Job drawing, mm, ordinate dimensions from the low corner. One solid piece. A direction names the side the tool comes from. Give positions to 0.01 mm unless a question says otherwise; leave off trailing zeros. Order: outer loops, then holes, each group sorted by start corner. A loop starts at its lowest first (then second) coordinate and runs counter-clockwise, first axis right, second up.
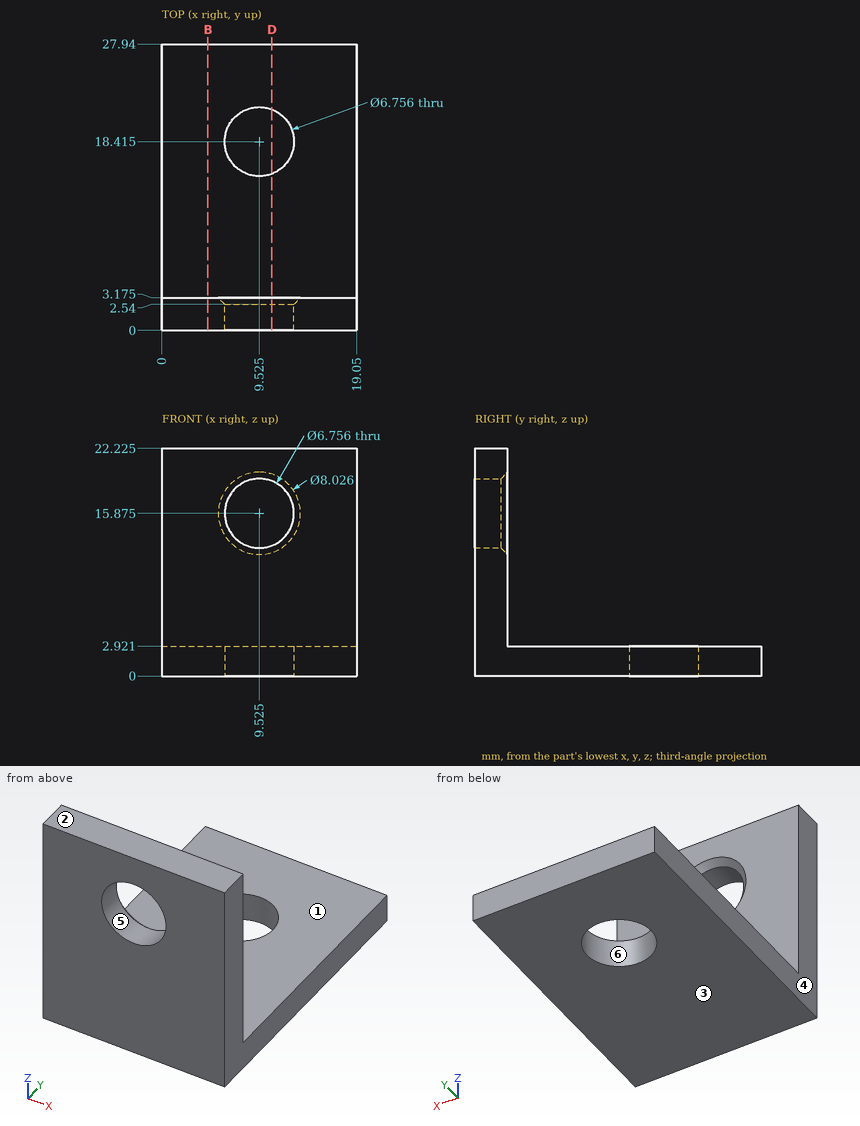
Item 1: Pull direction X, two halves, no side cores. Call the marked faces 3, 4, 5 and 6: released by +X, released by -X, zero draft, split by the parting line, or undercut.
Item 2: Drill centre lines: probe 1 along Z at (x, y) = (17, 18.75); probe 2 along Y at (x, z) = (1.5, 6) (1 decimal); probe 3 along X at (y, z) = (2.5, 13.5). Where is each one in solid material? Low to high.
Item 3: Drop flat-ended pins along their axis: P1, Ø4, axis at x = 4.5, y = 9, coming from the +Z side; P2, Ø6, axis at x = 9.525, y = 18.415, coming from the +Z side. Give the stop position or say it passes through.
Item 4: Band-saw the part on D-D on x = 10.75. Give the number of separate pieces and of enclosed holes in the cut face, plus the area to 3 significant figures.
Item 5: Which spindle directions (+Z, -Z, +X, -X, +Y, -Y) get a long thin tool onto all of the face, cutting with end or side? Do the marked faces 1 and 2. Say none if no direction does.
Item 6: Band-saw the part on B-B on x = 4.5. List the corners of the cut face in (y, z) (1 decimal), plus the area to 3 significant figures.
Working result:
1. face 3: zero draft
1. face 4: released by -X
1. face 5: undercut
1. face 6: undercut
2. probe 1: z = 0 to 2.92
2. probe 2: y = 0 to 3.2
2. probe 3: x = 0 to 7.12, 11.93 to 19.05
3. P1: stops at z = 2.92
3. P2: passes through
4. separate pieces: 3
4. enclosed holes: 0
4. area: 104 mm2
5. face 1: +Z, +X, -X, +Y
5. face 2: +Z, +X, -X, +Y, -Y
6. outline: (0, 0) - (27.9, 0) - (27.9, 2.9) - (3.2, 2.9) - (3.2, 22.2) - (0, 22.2) - close
6. area: 143 mm2
